Source: three-view drawing plus pictorial views. Frame: mm from the lowest corner of the part. A direction names the side the tool comes from. Give positions to 0.01 mm unless a question says otherwise; leave off trailing zeros. Loops run counter-clockwise (first coordinate to the right, second up) from the corner with the lowest first, then second, coordinate; pieces in that order, holes last. Notation, with made-up numbers: (60.5, 56.5) -> (99.5, 56.5) arc R22 ccw to (99.5, 63.5) -> close; hole circle Ø2 at (57.5, 23.5). An arc over 180 degrees is marked (long way). One line per item, written item: value. Start each with the question number.
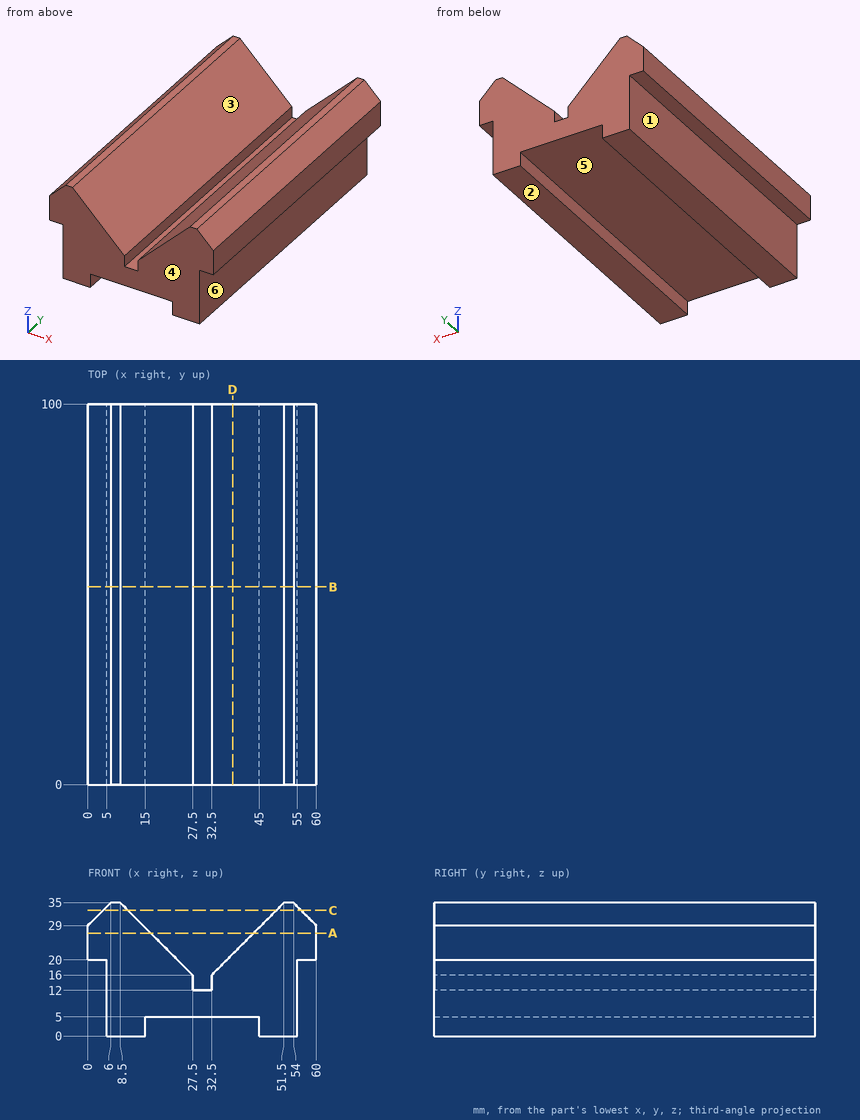
Item 1: Section A-A, the plane z = 27. Output: boundary loops of the cut face in (x, y).
Item 2: Section C-C, the plane z = 33. Output: boundary loops of the cut face in (x, y), then the cut area to 3 significant figures.
Item 3: Section D-D, the plane x = 38. Output: boundary loops of the cut face in (y, z).
Item 4: Pin query (flat end, axial travel): pin 1 (2.5 mm diameter, centred on y = 64.5, z = 1.5, fed in from -X); pin 2 (4 mm diameter, centred on x = 14.5, y = 71, fed in from +Z); pin 3 (2.5 mm diameter, centred on x = 56.5, y = 55.5, fed in from -Z). Return the tip coordinate at first contact, or that it passes through.
Item 5: Section B-B, the plane y = 52. Output: boundary loops of the cut face in (x, z), then the cut area to 3 significant figures.
Item 6: Mould query, pull axis X, two halves, no side actions, for the marked faces 3, 4, 5 and 6. Classes: pulls with the +X half, pulls with the -X half, needs draft (parallel to the pull), parting line crosses it, or undercut.
Item 7: Ray query, line 1 along X through (y, z) = (65, 2.5); line 2 along X through (y, z) = (75.5, 14); line 3 along X through (y, z) = (67, 10.5). Return the intervals inside material, ascending. Write a range as [from, to].
Item 8: Access query for the marked faces 1 and 2. Directions: +Z, -Z, +X, -X, +Y, -Y. A direction counts if a zero-diameter tool reaches every point of the face in a straight line with its end or side. Return the directions, or none.
Geometry check:
1. outline: (0, 0) -> (16.5, 0) -> (16.5, 100) -> (0, 100) -> close; (43.5, 0) -> (60, 0) -> (60, 100) -> (43.5, 100) -> close
2. outline: (4, 0) -> (10.5, 0) -> (10.5, 100) -> (4, 100) -> close; (49.5, 0) -> (56, 0) -> (56, 100) -> (49.5, 100) -> close
2. area: 1,300 mm2
3. outline: (0, 5) -> (100, 5) -> (100, 21.5) -> (0, 21.5) -> close
4. pin 1: stops at x = 5
4. pin 2: stops at z = 31
4. pin 3: stops at z = 20
5. outline: (0, 20) -> (5, 20) -> (5, 0) -> (15, 0) -> (15, 5) -> (45, 5) -> (45, 0) -> (55, 0) -> (55, 20) -> (60, 20) -> (60, 29) -> (54, 35) -> (51.5, 35) -> (32.5, 16) -> (32.5, 12) -> (27.5, 12) -> (27.5, 16) -> (8.5, 35) -> (6, 35) -> (0, 29) -> close
5. area: 1,240 mm2
6. face 3: undercut
6. face 4: needs draft
6. face 5: undercut
6. face 6: pulls with the +X half
7. line 1: x = [5, 15], [45, 55]
7. line 2: x = [5, 27.5], [32.5, 55]
7. line 3: x = [5, 55]
8. face 1: -Z, -X, +Y, -Y
8. face 2: -Z, +X, -X, +Y, -Y
